The figure shows three views and two pictorial views of one solid part (mm, origin at its lowest corner). Answer the questions. Give positions to 0.01 mm unless a question says otherwise; leave off trailing zeros. Loops run counter-clockwise (first coordinate to the right, second up) from the corner with the lowest first, then second, coordinate; pieces in that order, holes last. Notation, with made-up numbers: M 50,21 L 74,21 A21 ccw 74,36 Z; hole C 88,-5.75 d6. An arc over 180 degrees is marked long. Write item = value, one per line. Start each with the question number.
1. Consider L1, parallel to Y at x = 13, z = 2.7; L2, parallel to Y at x = 67, z = 4.1; L3, parallel to Y at x = 55.5, z = 4.2. Determine where each line is inside the solid, lowest interval first. Write a range as [from, to].
2. Section C-C on y = 87.5 is taken. Determine the outline of the cut face in (x, z) (3 decimals), plus the area to 3 significant figures.
3. Section B-B on x = 67 is taken. Determine the outline of the cut face in (y, z) (3 decimals).
4. Section A-A on y = 37 is taken. Determine the outline of the cut face in (x, z), plus the area to 3 significant figures.
5. Section D-D on x = 15 is taken. Determine the outline of the cut face in (y, z).
6. Flat-ended cylindrical pins translate along their axes: pin 1 Ø1.8 at (x, y) = (67.5, 86.5) entering from -Z; pin 2 Ø1 at (y, z) = (122, 0.5) entering from +X; pin 3 Ø3 at (y, z) = (54.5, 4) entering from -X; pin 4 Ø12 at (x, y) = (79, 105) entering from -Z. Find the tip coordinate at first contact, or state that the pin passes through.
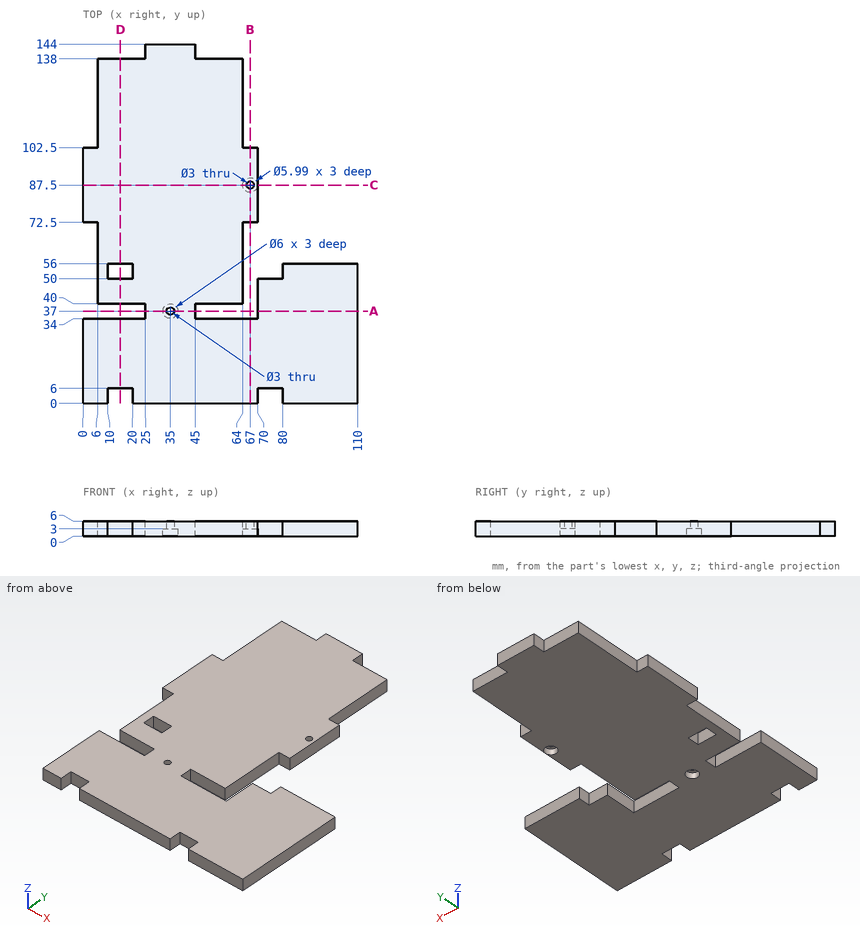
Verdict:
q1.L1 = [6, 34], [40, 50], [56, 138]
q1.L2 = [0, 34], [72.5, 86], [89, 102.5]
q1.L3 = [0, 34], [40, 138]
q2.outline = M 0,0 L 64.005,0 L 64.005,3 L 65.5,3 L 65.5,6 L 0,6 Z; M 68.5,3 L 69.995,3 L 69.995,0 L 70,0 L 70,6 L 68.5,6 Z
q2.area = 393 mm2
q3.outline = M 0,0 L 34,0 L 34,6 L 0,6 Z; M 72.5,0 L 84.505,0 L 84.505,3 L 86,3 L 86,6 L 72.5,6 Z; M 89,3 L 90.495,3 L 90.495,0 L 102.5,0 L 102.5,6 L 89,6 Z
q4.outline = M 25,0 L 32,0 L 32,3 L 33.5,3 L 33.5,6 L 25,6 Z; M 36.5,3 L 38,3 L 38,0 L 45,0 L 45,6 L 36.5,6 Z; M 70,0 L 110,0 L 110,6 L 70,6 Z
q4.area = 333 mm2
q5.outline = M 6,0 L 34,0 L 34,6 L 6,6 Z; M 40,0 L 50,0 L 50,6 L 40,6 Z; M 56,0 L 138,0 L 138,6 L 56,6 Z
q6.pin_1 = 3
q6.pin_2 = 64
q6.pin_3 = 6
q6.pin_4 = through
